Job drawing, mm, ordinate dimensions from the low corner. One solid piece. A direction names the side the tool comes from. Give positions to 0.01 mm unless a question says otherwise; leave off trailing zeros. Write each loop counter-clockwise with the first axis right and the second up, starting at its lowest first coordinate (ties: lowest second). Pieces come first, ordered by that corner, then holes. Notation, with made-up numbers: (2.5, 83) - (36.5, 83) arc R35 cw to (36.5, 120) - close; hole circle Ø8 at (64.25, 4). An arc over 180 degrees is marked (long way). Answer as a JSON object with one key per item and string values.
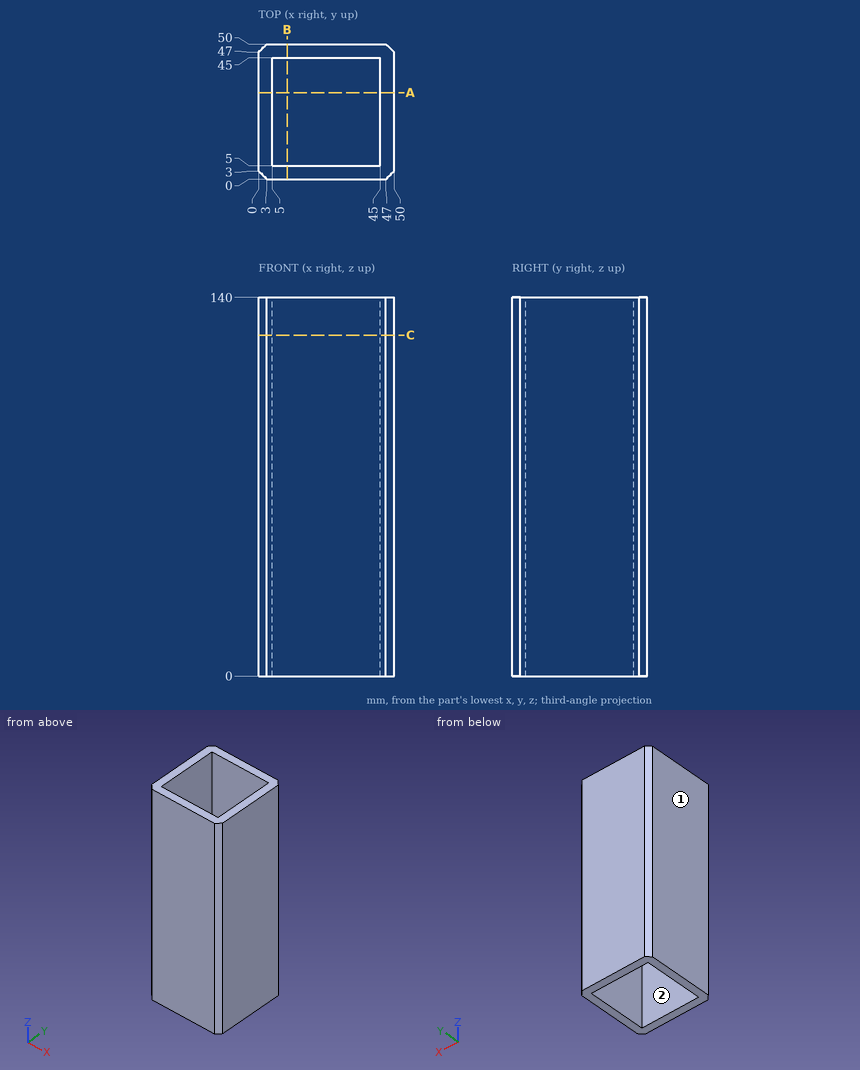
Item 1: Flat gauge pin, fed straight in: P1, Ø12, axis at y = 25, z = 41, coming from the -X side. Where does the tip first touch, or does it go through?
Entries:
{"P1": "x = 0"}
Item 2: Cut at A-A (y = 32). Give the cut face in (x, z).
Entries:
{"outline": "(0, 0) - (5, 0) - (5, 140) - (0, 140) - close; (45, 0) - (50, 0) - (50, 140) - (45, 140) - close"}
Item 3: Which spindle directions (+Z, -Z, +X, -X, +Y, -Y) get a long thin tool onto all of the face, cutting with end or side? Do the marked faces 1 and 2. Say none if no direction does.
Entries:
{"face 1": "+Z, -Z, -X, +Y, -Y", "face 2": "+Z, -Z"}
Item 4: Cut at C-C (z = 126). Give the cut face in (x, y).
Entries:
{"outline": "(0, 3) - (3, 0) - (47, 0) - (50, 3) - (50, 47) - (47, 50) - (3, 50) - (0, 47) - close; hole (5, 5) - (45, 5) - (45, 45) - (5, 45) - close"}
Item 5: Probe line 1 (Y direction, x = 37.5, z = 116); line 2 (X direction, y = 2, z = 28). List the from-to ranges inside material, lowest first. Write a range as from..to.
Entries:
{"line 1": "0..5, 45..50", "line 2": "1..49"}
